Source: CAD feature listing. Evaluate the final solid. Frame: model axes, mm. A direction names the side the tool comes from. Round coordinates to 2 decimals unless told otherwise and drop trailing zeros. Order: outer loops, then holes, each group sorted by start corner. A loop starts at its lowest first (then second) coordinate and runs counter-clockwise, first axis right, second up. Notation, with made-up numbers: (-4, 1) - (41, 1) arc R19 cw to (41, 26) - close; hole circle Ø4 at (59, 75.25). An arc over 180 degrees is marked (long way). Put each result on its own line as item: value. Start each with the question number.
1) Access query for faces 5 (the face through (24, 6, -20)), 6 (the face through (36.57, 13.49, -16.6)), 7 (the face through (36, 7, 1)), 8 (the face through (-0.5, 9.1, -4)), 9 (the face through (0, 6, -10)). Directions: +Z, -Z, +X, -X, +Y, -Y. A direction counts if a zero-diameter tool reaches every point of the face in a straight line with its end or side. Return the directions, or none.
2) Section B-B on z = -10. Output: boundary loops of the cut face in (x, y).
3) Contact query for flat-ended pins moving along their axis: P1, Ø4, axis at x = 26, y = 12.5, coming from the -Z side; P2, Ø6, axis at x = 40, z = 3, coming from the -Y side; P3, Ø8, axis at y = 7.5, z = -13, coming from the +X side; P4, Ø3.5, axis at x = 1.5, y = 6.5, coming from the -Z side. Output: stop coordinate, or through.
4) Section C-C on x = 24. Output: boundary loops of the cut face in (y, z).
5) Section A-A on y = 8. Output: boundary loops of the cut face in (x, z).
6) Line query: probe 1 along X at (y, z) = (1.3, -10); probe 2 along X at (y, z) = (12.75, -10); probe 3 along Z at (x, y) = (23.5, 12). Output: solid intervals per line, ascending. Write a range as [from, to].
7) Mould query, pull axis X, two halves, no side actions, for faces 1 (the face through (-3, 8, -10)), 2 (the face through (48, 6, -10)), 3 (the face through (24, 13, -10)), 4 (the face through (24, 7, 3)). Classes: +X half, -X half, draft (parallel to the pull), parting line (faces both ways), or undercut.
8) Section D-D on x = 42. Output: boundary loops of the cut face in (y, z), then the cut area to 3 significant figures.
```python
from build123d import *

# Parameters (mm, degrees)
SKETCH1_W           = 54
SKETCH1_H           = 26
SKETCH1_W_2         = 48
SKETCH1_H_2         = 20
BOSS_EXTRUDE1_DEPTH = 13
SKETCH2_W           = 54
SKETCH2_H           = 26
BOSS_EXTRUDE2_DEPTH = 2
SKETCH3_W           = 15
SKETCH3_H           = 7
CUT_EXTRUDE1_DEPTH  = 58.92236183
FILLET1_R           = 2
FILLET2_R           = 1
SKETCH4_R           = 1
BOSS_EXTRUDE3_DEPTH = 2
FILLET3_R           = 2


with BuildPart() as part:
    # Sketch1 → Boss-Extrude1 (new body)
    with BuildSketch(Plane(origin=(0, 0, 0), x_dir=(1, 0, 0), z_dir=(0, 1, 0))):
        with Locations((24, 10)):
            Rectangle(SKETCH1_W, SKETCH1_H)
        with Locations((24, 10)):
            Rectangle(SKETCH1_W_2, SKETCH1_H_2, mode=Mode.SUBTRACT)
    extrude(amount=BOSS_EXTRUDE1_DEPTH)

    # Sketch2 → Boss-Extrude2 (add)
    with BuildSketch(Plane(origin=(0, 13, 0), x_dir=(1, 0, 0), z_dir=(0, 1, 0))):
        with Locations((24, 10)):
            Rectangle(SKETCH2_W, SKETCH2_H)
    extrude(amount=BOSS_EXTRUDE2_DEPTH)

    # Sketch3 → Cut-Extrude1 (cut, through all)
    with BuildSketch(Plane(origin=(0, 15, 0), x_dir=(1, 0, 0), z_dir=(0, 1, 0))):
        with Locations((4.5, 19.5)):
            Rectangle(SKETCH3_W, SKETCH3_H)
        with Locations((4.5, 0.5)):
            Rectangle(SKETCH3_W, SKETCH3_H)
        with Locations((43.5, 0.5)):
            Rectangle(SKETCH3_W, SKETCH3_H)
        with Locations((43.5, 19.5)):
            Rectangle(SKETCH3_W, SKETCH3_H)
    extrude(amount=-CUT_EXTRUDE1_DEPTH, mode=Mode.SUBTRACT)

    # Fillet1
    fillet1_edges = [part.edges().sort_by_distance(p)[0] for p in [
        (12, 14, -16),
        (36, 14, -16),
        (36, 14, -4),
        (12, 14, -4),
    ]]
    fillet(fillet1_edges, radius=FILLET1_R)

    # Fillet2
    fillet2_edges = [part.edges().sort_by_distance(p)[0] for p in [
        (-3, 7.5, -16),
        (12, 7.5, -23),
        (3.5, 15, -16),
        (36, 15, 0.5),
        (3.5, 15, -4),
        (12, 15, -20.5),
        (44.5, 15, -16),
        (36.585786438, 15, -3.414213562),
        (11.414213562, 15, -3.414213562),
        (11.414213562, 15, -16.585786438),
        (36.585786438, 15, -16.585786438),
        (-3, 15, -10),
        (24, 15, 3),
        (51, 15, -10),
        (24, 15, -23),
        (51, 7.5, -16),
        (36, 7.5, -23),
        (36, 15, -20.5),
        (51, 7.5, -4),
        (36, 7.5, 3),
        (44.5, 15, -4),
        (-3, 7.5, -4),
        (12, 7.5, 3),
        (12, 15, 0.5),
    ]]
    fillet(fillet2_edges, radius=FILLET2_R)

    # Sketch4 → Boss-Extrude3 (add)
    # profile 1 of 4: a face of its own
    with BuildSketch(Plane.XZ):
        with BuildLine():
            Line((24, 3), (21, 3))
            Line((21, 3), (21, 6))
            ThreePointArc((21, 6), (21.585786438, 7.414213562), (23, 8))
            Line((23, 8), (25, 8))
            ThreePointArc((25, 8), (26.414213562, 7.414213562), (27, 6))
            Line((27, 6), (27, 3))
            Line((27, 3), (24, 3))
        make_face()
        with Locations(Location((24, 5.034061628, 0), (0, 0, 270))):
            Circle(SKETCH4_R, mode=Mode.SUBTRACT)
    # profile 2 of 4: a face of its own
    with BuildSketch(Plane.XZ):
        with BuildLine():
            Line((27, -23), (24, -23))
            Line((24, -23), (21, -23))
            Line((21, -23), (21, -26))
            ThreePointArc((21, -26), (21.585786438, -27.414213562), (23, -28))
            Line((23, -28), (25, -28))
            ThreePointArc((25, -28), (26.414213562, -27.414213562), (27, -26))
            Line((27, -26), (27, -23))
        make_face()
        with Locations(Location((24, -25.034061628, 0), (0, 0, 90))):
            Circle(SKETCH4_R, mode=Mode.SUBTRACT)
    # profile 3 of 4: a face of its own
    with BuildSketch(Plane.XZ):
        with BuildLine():
            Line((-3, -10), (-3, -7))
            Line((-3, -7), (-6, -7))
            ThreePointArc((-6, -7), (-7.414213562, -7.585786438), (-8, -9))
            Line((-8, -9), (-8, -11))
            ThreePointArc((-8, -11), (-7.414213562, -12.414213562), (-6, -13))
            Line((-6, -13), (-3, -13))
            Line((-3, -13), (-3, -10))
        make_face()
        with Locations(Location((-5.274023851, -10, 0), (0, 0, 270))):
            Circle(SKETCH4_R, mode=Mode.SUBTRACT)
    # profile 4 of 4: a face of its own
    with BuildSketch(Plane.XZ):
        with BuildLine():
            Line((51, -13), (51, -10))
            Line((51, -10), (51, -7))
            Line((51, -7), (54, -7))
            ThreePointArc((54, -7), (55.414213562, -7.585786438), (56, -9))
            Line((56, -9), (56, -11))
            ThreePointArc((56, -11), (55.414213562, -12.414213562), (54, -13))
            Line((54, -13), (51, -13))
        make_face()
        with Locations(Location((53.274023851, -10, 0), (0, 0, 90))):
            Circle(SKETCH4_R, mode=Mode.SUBTRACT)
    extrude(amount=-BOSS_EXTRUDE3_DEPTH)

    # Fillet3
    fillet3_edges = [part.edges().sort_by_distance(p)[0] for p in [
        (27, 1, 3),
        (21, 1, 3),
        (51, 1, -7),
        (51, 1, -13),
        (27, 1, -23),
        (21, 1, -23),
        (-3, 1, -13),
        (-3, 1, -7),
    ]]
    fillet(fillet3_edges, radius=FILLET3_R - 0.0001)  # a hair under: the kernel refuses the full size


solid = part.part
```
Answer sheet:
1. face 5: +X, -X, -Y
1. face 6: -Z, +X, +Y, -Y
1. face 7: +Z, +X, +Y, -Y
1. face 8: +Z, -X, +Y, -Y
1. face 9: +Z, -Z, -Y
2. outline: (-8, 0) - (-6.27, 0) - (-6.27, 2) - (-8, 2) - close; (-4.27, 0) - (0, 0) - (0, 13) - (48, 13) - (48, 0) - (52.27, 0) - (52.27, 2) - (51, 2) - (51, 14) arc R1 ccw to (50, 15) - (-2, 15) arc R1 ccw to (-3, 14) - (-3, 2) - (-4.27, 2) - close; (54.27, 0) - (56, 0) - (56, 2) - (54.27, 2) - close
3. P1: z = -23
3. P2: through
3. P3: x = 51
3. P4: z = -16
4. outline: (0, -28) - (2, -28) - (2, -26.03) - (0, -26.03) - close; (0, -24.03) - (2, -24.03) - (2, -23) - (14, -23) arc R1 ccw to (15, -22) - (15, 2) arc R1 ccw to (14, 3) - (2, 3) - (2, 4.03) - (0, 4.03) - (0, 0) - (13, 0) - (13, -20) - (0, -20) - close; (0, 6.03) - (2, 6.03) - (2, 8) - (0, 8) - close
5. outline: (-3, -15) arc R1 ccw to (-2, -16) - (0, -16) - (0, -4) - (-2, -4) arc R1 ccw to (-3, -5) - close; (12, -22) arc R1 ccw to (13, -23) - (35, -23) arc R1 ccw to (36, -22) - (36, -20) - (12, -20) - close; (12, 0) - (36, 0) - (36, 2) arc R1 ccw to (35, 3) - (13, 3) arc R1 ccw to (12, 2) - close; (48, -16) - (50, -16) arc R1 ccw to (51, -15) - (51, -5) arc R1 ccw to (50, -4) - (48, -4) - close
6. probe 1: [-8, -6.27], [-4.27, 0], [48, 52.27], [54.27, 56]
6. probe 2: [-3, 0], [48, 51]
6. probe 3: [-23, -20], [0, 3]
7. face 1: -X half
7. face 2: undercut
7. face 3: undercut
7. face 4: draft
8. outline: (13, -16) - (14, -16) arc R1 ccw to (15, -15) - (15, -5) arc R1 ccw to (14, -4) - (13, -4) - close
8. area: 23.6 mm^2
